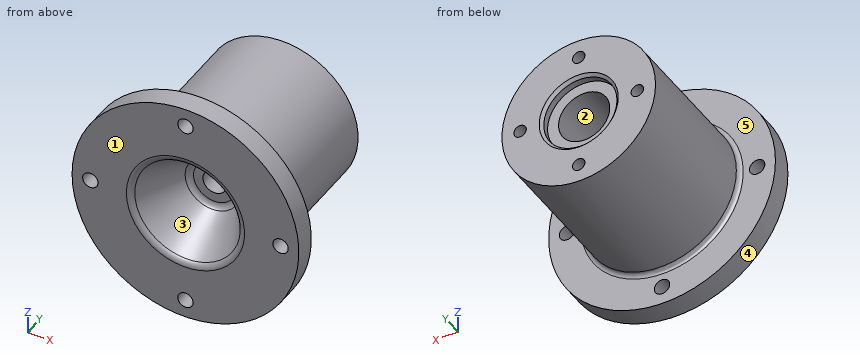
from build123d import *

# Parameters (mm, degrees)
FILLET1_R                    = 3
FILLET2_R                    = 5
FILLET3_R                    = 2.5
CHAMFER1_SIZE                = 2
M10_CLEARANCE_HOLE2_D        = 10.5
R_P_TITION_CIRCULAIRE1_COUNT = 4


with BuildPart() as part:
    # Sketch2 → Revolve1 (revolve)
    with BuildSketch(Plane.XY, mode=Mode.PRIVATE) as revolve1_sk:
        with BuildLine():
            Line((25, 115), (25, 108.5))
            Line((25, 108.5), (17.5, 108.5))
            Line((17.5, 108.5), (17.5, 51))
            Line((17.5, 51), (8, 51))
            Line((8, 51), (8, 35))
            Line((8, 35), (14.405989232, 35))
            ThreePointArc((14.405989232, 35), (16.905989232, 34.330127019), (18.736116251, 32.5))
            Line((18.736116251, 32.5), (37.5, 0))
            Line((37.5, 0), (77.5, 0))
            Line((77.5, 0), (77.5, 15))
            Line((77.5, 15), (52.5, 15))
            Line((52.5, 15), (52.5, 115))
            Line((52.5, 115), (25, 115))
        make_face()
    revolve(revolve1_sk.sketch.rotate(Axis((0, -0.774116112, 0), (0, -1, 0)), 180), axis=Axis((0, -0.774116112, 0), (0, -1, 0)))

    # Fillet1
    fillet1_edges = [part.edges().sort_by_distance(p)[0] for p in [
        (52.5, 15, 0),
    ]]
    fillet(fillet1_edges, radius=FILLET1_R)

    # Fillet2
    fillet2_edges = [part.edges().sort_by_distance(p)[0] for p in [
        (37.5, 0, 0),
    ]]
    fillet(fillet2_edges, radius=FILLET2_R)

    # Fillet3
    fillet3_edges = [part.edges().sort_by_distance(p)[0] for p in [
        (17.5, 51, 0),
    ]]
    fillet(fillet3_edges, radius=FILLET3_R)

    # Chamfer1
    chamfer1_edges = [part.edges().sort_by_distance(p)[0] for p in [
        (25, 115, 0),
    ]]
    chamfer(chamfer1_edges, length=CHAMFER1_SIZE)

    # M10 Clearance Hole2 (through all)
    with Locations(Plane(origin=(0, 15, 0), x_dir=(1, 0, 0), z_dir=(0, 1, 0))):
        with Locations((0, 65), (65, 0), (0, -65), (-65, 0)):
            Hole(M10_CLEARANCE_HOLE2_D / 2)

    # Esquisse5 → Trou taraudé M101 (revolve, cut)
    with BuildSketch(Plane(origin=(-40.072621641, 115, 0), x_dir=(0, 0, 1), z_dir=(1, 0, 0))):
        Polygon((0, 0), (0, 30.053657631), (4.25, 27.5), (4.25, 0), align=None)
    trou_taraud_m101 = revolve(axis=Axis((-40.072621641, 121.35, 0), (0, -1, 0)), mode=Mode.SUBTRACT)

    # Répétition circulaire1: Trou taraudé M101 ×4 about axis
    r_p_tition_circulaire1_axis = Axis((0, 0, 0), (0, 1, 0))
    for i in range(1, R_P_TITION_CIRCULAIRE1_COUNT):
        add(trou_taraud_m101.rotate(r_p_tition_circulaire1_axis, i * 360 / R_P_TITION_CIRCULAIRE1_COUNT), mode=Mode.SUBTRACT)


solid = part.part
Geometry: final body of the model. Coordinates: model frame, mm. Face numbers are marked on the shaded views. A direction names the side the tool comes from. Coordinates: 2 decimals unless noted, no trailing zeros. Loops run counter-clockwise (first coordinate to the right, second up) from the corner with the lowest first, then second, coordinate; pieces in that order, holes last. Notation, with made-up numbers: M -34,-31 L 10,-31 A22 ccw 10,6 Z; hole C 15,19 d9. An arc over 180 degrees is marked long. One line per item, written item: value. Start each with the question number.
1) Draft query along Z for the marked faces 3, 4 and 5. Return one class per face: released by +Z, released by -Z, zero draft, split by the parting line, or undercut.
2) Cut plane A-A (z = -65). Return loops of the section in (x, y), then the cut area to 3 significant figures.
3) Material intervals for L1, parallel to Z at x = 0, y = 111; L2, parallel to Z at x = 0, y = 12.25; L3, parallel to Y at x = 8.5, z = 70.5, sorted ascending. Write a range as from..to.
4) Cut plane C-C (y = 94.5). Return loops of the section in (x, z), then the cut area to 3 significant figures.
5) Cut plane B-B (x = 65). Return loops of the section in (y, z).
6) Cut plane D-D (y = 13). Return loops of the section in (x, z).
7) Pin query (flat end, axial travel): P1, Ø13.5, axis at x = 0, z = -65, coming from the +Y side; P2, Ø10, axis at y = 32, z = -22, coming from the -X side; P3, Ø4, axis at x = -8.5, z = 36, coming from the -Y side; P4, Ø6.5, axis at x = -65, z = 0, coming from the +Y side. Return the tip coordinate at first contact, or that it passes through.
8) Reachability of the marked faces 1 and 2 from +Z, -Z, +X, -X, +Y, -Y: full face, straight path, thin tool, end or side. Return the list, or none.
Evaluation:
1. face 3: undercut
1. face 4: split by the parting line
1. face 5: zero draft
2. outline: M -42.2,0 L -5.25,0 L -5.25,15 L -42.2,15 Z; M 5.25,0 L 42.2,0 L 42.2,15 L 5.25,15 Z
2. area: 1,110 mm^2
3. L1: -52.5..-44.32, -35.82..-25, 25..35.82, 44.32..52.5
3. L2: -77.5..-70.25, -59.75..-30.43, 30.43..59.75, 70.25..77.5
3. L3: 0..15
4. outline: C 0,0 d105; hole C -40.07,0 d8.5; hole C 0,0 d35; hole C 0,-40.07 d8.5; hole C 0,40.07 d8.5; hole C 40.07,0 d8.5
4. area: 7,470 mm^2
5. outline: M 0,-42.2 L 15,-42.2 L 15,-5.25 L 0,-5.25 Z; M 0,5.25 L 15,5.25 L 15,42.2 L 0,42.2 Z
6. outline: C 0,0 d155; hole C -65,0 d10.5; hole C 0,0 d59.99; hole C 0,-65 d10.5; hole C 0,65 d10.5; hole C 65,0 d10.5
7. P1: y = 15
7. P2: x = -49.67
7. P3: y = 0.2
7. P4: through
8. face 1: +Z, -Z, +X, -X, -Y
8. face 2: +Y
